Build history of the part. All positions in model axes, mm. Face numbers are marked on the shaded views. A direction names the side the tool comes from. Round coordinates to 2 decimals unless told otherwise and drop trailing zeros. Loops run counter-clockwise (first coordinate to the right, second up) from the corner with the lowest first, then second, coordinate; pieces in that order, holes last. Notation, with made-up numbers: (-24, 24.25) - (34, 24.25) arc R8 ccw to (34, 37.25) - close; hole circle Ø1 at (35.25, 33). An arc over 180 degrees is marked (long way). Put each result on its own line as item: value. Start each with the question number.
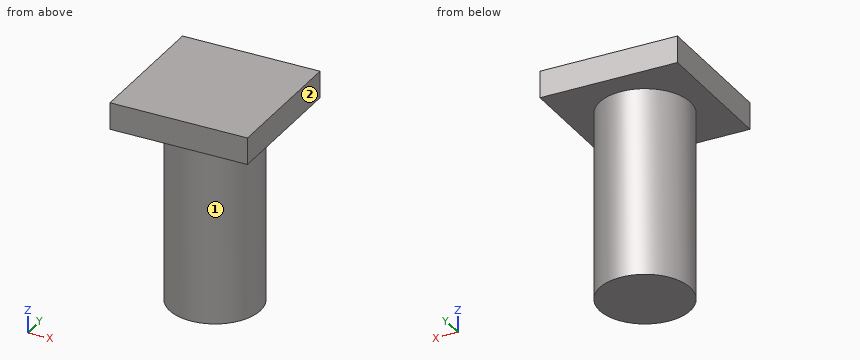
from build123d import *

# Parameters (mm, degrees)
SKETCH1_R           = 16.892448346
BOSS_EXTRUDE1_DEPTH = 70
SKETCH2_W           = 51.249127752
SKETCH2_H           = 51.249127751
BOSS_EXTRUDE2_DEPTH = 10


with BuildPart() as part:
    # Sketch1 → Boss-Extrude1 (new body)
    with BuildSketch(Plane.XY):
        with Locations((-8.123318292, -5.927826862)):
            Circle(SKETCH1_R)
    extrude(amount=BOSS_EXTRUDE1_DEPTH)

    # Sketch2 → Boss-Extrude2 (add)
    with BuildSketch(Plane.XY.offset(70)):
        with Locations((-8.123318292, -5.927826862)):
            Rectangle(SKETCH2_W, SKETCH2_H)
    extrude(amount=BOSS_EXTRUDE2_DEPTH)


solid = part.part
1) Slice it at D-D, the plane x = 12. Write the cut outline in (y, z).
2) Drill centre lines: line 1 (Z direction, x = 14.5, y = -17); line 2 (Y direction, x = 2, z = 47); line 3 (Y direction, x = -4.5, z = 41). Where is each one in solid material? Low to high. Write a range as [from, to].
3) Slice it at B-B, the plane y = -4.5. Write the cut outline in (x, z), and give its area (3 significant figures).
4) Slice it at C-C, the plane z = 6. Write the cut outline in (x, y).
5) Drop flat-ended pins along their axis: pin 1 Ø6 at (x, z) = (-0.5, 54) entering from +Y; pin 2 Ø6 at (x, z) = (-23, 41) entering from -Y; pin 3 Ø6 at (y, z) = (-8, 61) entering from -X. Give the stop position or say it passes through.
6) Which spindle directions (+Z, -Z, +X, -X, +Y, -Y) get a long thin tool onto all of the face, cutting with end or side? Do the marked faces 1 and 2. Say none if no direction does.
7) Slice it at A-A, the plane x = -13. Write the cut outline in (y, z).
Taken from the geometry:
1. outline: (-31.55, 70) - (19.7, 70) - (19.7, 80) - (-31.55, 80) - close
2. line 1: z = [70, 80]
2. line 2: y = [-19.45, 7.6]
2. line 3: y = [-22.43, 10.57]
3. outline: (-33.75, 70) - (-24.96, 70) - (-24.96, 0) - (8.71, 0) - (8.71, 70) - (17.5, 70) - (17.5, 80) - (-33.75, 80) - close
3. area: 2,870 mm2
4. outline: circle Ø33.78 at (-8.12, -5.93)
5. pin 1: stops at y = 10.32
5. pin 2: stops at y = -17.94
5. pin 3: stops at x = -25.02
6. face 1: -Z
6. face 2: +Z, -Z, +X, +Y, -Y
7. outline: (-31.55, 70) - (-22.1, 70) - (-22.1, 0) - (10.25, 0) - (10.25, 70) - (19.7, 70) - (19.7, 80) - (-31.55, 80) - close
